Part model, mm, in its own coordinate system. A direction names the side the tool comes from. Coordinates: 2 decimals unless noted, no trailing zeros. Loops run counter-clockwise (first coordinate to the right, second up) from the corner with the lowest first, then second, coordinate; pieces in that order, holes last. Notation, with made-up numbers: (20.25, -32) - (68.25, -32) arc R34 ccw to (68.25, -2) - close; hole circle Ø9 at (-19, 20). An arc over 180 degrees is marked (long way). Use a Markdown table: item, result. Add a question column.
1) Tool access for faces 4 (the face through (0, 92, -7)), 5 (the face through (0.47, 71.79, -13.49)): list every direction of +Z, -Z, +X, -X, +Y, -Y with a clear straight run to the whole face (end or side of a thin tool).
2) Band-saw the part on A-A (z = 0). Give the cut face in (x, y).
3) Band-saw the part on C-C (z = -15). Give the cut face in (x, y), plus the area to 3 significant figures.
4) Band-saw the part on B-B (x = 1). Give the cut face in (y, z).
5) Drop flat-ended pins along their axis: P1, Ø2, axis at y = 78.5, z = -11, coming from the -X side; P2, Ø10, axis at x = 22, z = -16, coming from the -Y side; P3, Ø1.5, axis at x = -1, y = 69.5, coming from the -Z side; P4, Ø5, axis at y = 10, z = 0, coming from the -X side. Give the stop position or say it passes through.
6) Probe probe 1 along Y at (x, z) = (6, 0); probe 2 along Y at (x, z) = (-12, -19); probe 3 along X at (y, z) = (39, -0.5). List the from-to ranges inside material, lowest first. Write a range as [from, to].
7) Pull direction Y, two halves, no side cores. Call faces 1 (the face through (0, 78, 10.5)), 2 (the face through (-0.14, 13.222, 0.423)), 3 (the face through (0, 0, 0)): +Y half, -Y half, draft (parallel to the pull), parting line (faces both ways), or undercut.
8) Band-saw the part on D-D (x = 12). Give the cut face in (y, z).
from build123d import *

# Parameters (mm, degrees)
SKETCH_1_R               = 10
EXTRUDE_1_DEPTH          = 57
SKETCH_2_R               = 13.5
EXTRUDE_2_DEPTH          = 30
CUT_EXTRUDE_1_DEPTH      = 90.070197036
CUT_EXTRUDE_1_DEPTH_BACK = 90.070197036
SKETCH_7_R               = 3.25
SKETCH_8_W               = 27
SKETCH_8_H               = 6
CUT_EXTRUDE_2_DEPTH      = 90.070197133
SKETCH_9_W               = 65
SKETCH_9_H               = 35
EXTRUDE_3_DEPTH          = 5


with BuildPart() as part:
    # 스케치1 → 보스-돌출1 (new body)
    with BuildSketch(Plane(origin=(0, 0, 0), x_dir=(1, 0, 0), z_dir=(0, 1, 0))):
        with Locations(Location((0, 0, 0), (0, 0, 90))):
            Circle(SKETCH_1_R)
    extrude(amount=EXTRUDE_1_DEPTH)

    # 스케치2 → 보스-돌출2 (add)
    with BuildSketch(Plane(origin=(0, 57, 0), x_dir=(1, 0, 0), z_dir=(0, 1, 0))):
        with Locations(Location((0, 0, 0), (0, 0, 270))):
            Circle(SKETCH_2_R)
    extrude(amount=EXTRUDE_2_DEPTH)

    # 스케치7 → 컷-돌출1 (cut, two sides: drawn at the far end of the back side and taken through both)
    with BuildSketch(Plane(origin=(0, 0, 0), x_dir=(0, 0, -1), z_dir=(1, 0, 0)).offset(-CUT_EXTRUDE_1_DEPTH_BACK)):
        with Locations((0, 10)):
            Circle(SKETCH_7_R)
    extrude(amount=CUT_EXTRUDE_1_DEPTH + CUT_EXTRUDE_1_DEPTH_BACK, mode=Mode.SUBTRACT)

    # 스케치8 → 컷-돌출2 (cut, through all)
    with BuildSketch(Plane(origin=(0, 87, 0), x_dir=(1, 0, 0), z_dir=(0, 1, 0))):
        with Locations((0, -13.5)):
            Rectangle(SKETCH_8_W, SKETCH_8_H)
    extrude(amount=-CUT_EXTRUDE_2_DEPTH, mode=Mode.SUBTRACT)

    # 스케치9 → 보스-돌출3 (add)
    with BuildSketch(Plane(origin=(0, 87, 0), x_dir=(1, 0, 0), z_dir=(0, 1, 0))):
        with Locations((0, 7)):
            Rectangle(SKETCH_9_W, SKETCH_9_H)
    extrude(amount=EXTRUDE_3_DEPTH)


solid = part.part
Answer block:
| question | item | result |
|---|---|---|
| 1 | face 4 | +Z, -Z, +X, -X, +Y |
| 1 | face 5 | -Y |
| 2 | outline | (-32.5, 87) - (-13.5, 87) - (-13.5, 57) - (-10, 57) - (-10, 13.25) - (10, 13.25) - (10, 57) - (13.5, 57) - (13.5, 87) - (32.5, 87) - (32.5, 92) - (-32.5, 92) - close; (-10, 0) - (10, 0) - (10, 6.75) - (-10, 6.75) - close |
| 3 | outline | (-32.5, 87) - (32.5, 87) - (32.5, 92) - (-32.5, 92) - close |
| 3 | area | 325 mm2 |
| 4 | outline | (0, -9.95) - (57, -9.95) - (57, -13.46) - (87, -13.46) - (87, -24.5) - (92, -24.5) - (92, 10.5) - (57, 10.5) - (57, 9.95) - (0, 9.95) - close; hole circle Ø6.5 at (10, 0) |
| 5 | P1 | x = -9.07 |
| 5 | P2 | y = 87 |
| 5 | P3 | z = -13.5 |
| 5 | P4 | through |
| 6 | probe 1 | [0, 6.75], [13.25, 92] |
| 6 | probe 2 | [87, 92] |
| 6 | probe 3 | [-9.99, 9.99] |
| 7 | face 1 | draft |
| 7 | face 2 | undercut |
| 7 | face 3 | -Y half |
| 8 | outline | (57, -6.18) - (87, -6.18) - (87, -24.5) - (92, -24.5) - (92, 10.5) - (87, 10.5) - (87, 6.18) - (57, 6.18) - close |
